```python
from build123d import *

# Parameters (mm, degrees)
FILLET_1_R  = 0.1
HEX_2_DEPTH = 1.04


with BuildPart() as part:
    # Эскиз1 → Body (revolve)
    with BuildSketch(Plane.XY):
        with BuildLine():
            Line((0, 1.425), (0, 0))
            Line((0, 0), (17.65, 0))
            Line((17.65, 0), (17.65, 1.2195))
            Line((17.65, 1.2195), (17.3695, 1.5))
            Line((17.3695, 1.5), (1.65, 1.5))
            Line((1.65, 1.5), (1.65, 2.85))
            Line((1.65, 2.85), (1.271128829, 2.85))
            ThreePointArc((1.271128829, 2.85), (0.531880191, 2.229988425), (0, 1.425))
        make_face()
    revolve(axis=Axis((-3.643489966, 0, 0), (-1, 0, 0)))

    # Скругление1
    fillet_1_edges = [part.edges().sort_by_distance(p)[0] for p in [
        (1.65, -1.5, 0),
    ]]
    fillet(fillet_1_edges, radius=FILLET_1_R)

    # Эскиз2 → Вырез-Повернуть1 (revolve, cut)
    with BuildSketch(Plane.XY):
        Polygon((0, 0), (0, 1), (1.04, 1), (1.617350269, 0), align=None)
    revolve(axis=Axis((1.617350269, 0, 0), (-1, 0, 0)), mode=Mode.SUBTRACT)

    # Эскиз3 → Hex 2 (cut)
    with BuildSketch(Plane.ZY):
        Polygon((-1, -0.577350269), (0, -1.154700538), (1, -0.577350269), (1, 0.577350269), (0, 1.154700538), (-1, 0.577350269), align=None)
    extrude(amount=-HEX_2_DEPTH, mode=Mode.SUBTRACT)


solid = part.part
```
Build history of the part. All positions in model axes, mm. A direction names the side the tool comes from. Give positions to 0.01 mm unless a question says otherwise; leave off trailing zeros. Loops run counter-clockwise (first coordinate to the right, second up) from the corner with the lowest first, then second, coordinate; pieces in that order, holes last.
Item 1: Slice it at A-A, the plane x = 9.5. List the corners of the cut face in (y, z).
Answers follow:
outline: circle Ø3 at (0, 0)
Item 2: Pull direction Y, two halves, no side cores. Call faces 1 (the face through (17.65, 0, 0)), 2 (the face through (0.51, -0.87, 0.49)), 3 (the face through (9.45, -1.5, -0.07)): released by +Y, released by -Y, zero draft, split by the parting line, or undercut.
Answers follow:
face 1: zero draft
face 2: undercut
face 3: split by the parting line
Item 3: Slice it at C-C, the plane z = 1.9. List the corners of the cut face in (x, y), and give its area (3 significant figures).
Answers follow:
outline: (1.27, -2.12) - (1.65, -2.12) - (1.65, 2.12) - (1.27, 2.12) arc R2.76 ccw to start
area: 4.56 mm2
Item 4: Flat gauge pin, fed straight in: pin 1 (2 mm diameter, centred on x = 14, y = -1, fed in from +Z). Where does the tip first touch, or does it go through?
Answers follow:
pin 1: stops at z = 1.5
Item 5: Which spindle directions (+Z, -Z, +X, -X, +Y, -Y) get a long thin tool onto all of the face, cutting with end or side? Do faces 4 (the face through (1.458, -2.262, 1.734)), 5 (the face through (1.65, 0, 2)), 6 (the face through (0.5, 0, -1)). Say none if no direction does.
Answers follow:
face 4: +X, -X
face 5: +X
face 6: -X
Item 6: Drill centre lines: line 1 (Z direction, x = 6.25, y = -0.1); line 2 (X direction, y = 1.45, z = 2.1); line 3 (X direction, y = 0.25, z = -2.05). Where is each one in solid material? Low to high.
Answers follow:
line 1: z = -1.5 to 1.5
line 2: x = 0.86 to 1.65
line 3: x = 0.39 to 1.65
Item 7: Slice it at B-B, the plane y = -2.25. List the corners of the cut face in (x, z), and give its area (3 significant figures).
Answers follow:
outline: (1.27, -1.75) - (1.65, -1.75) - (1.65, 1.75) - (1.27, 1.75) arc R2.48 ccw to start
area: 3.06 mm2
